For this review, take the finished solid that the model builds, in its own axes (mm). Face numbers are marked on the shaded views. A direction names the side the tool comes from. Give positions to 0.01 mm unless a question says otherwise; leave off trailing zeros. Order: outer loops, then holes, each group sorted by start corner. A loop starts at its lowest first (then second) coordinate and runs counter-clockwise, first axis right, second up.
Autodesk Inventor part; units mm, degrees
ref_plane "YZ Plane" through (0, 0, 0) normal (1, 0, 0) x (0, 1, 0)
ref_plane "XZ Plane" through (0, 0, 0) normal (0, 1, 0) x (-1, 0, 0)
ref_plane "XY Plane" through (0, 0, 0) normal (0, 0, 1) x (1, 0, 0)
sketch "Sketch1" plane through (0, 0, 0) normal (0, 0, 1) x (1, 0, 0)
  circle A0 centre (0, 0) radius 8.4
  circle A1 centre (0, 0) radius 11
  line L0 (9.5093, -0.878) -> (0, 0)
  line L1 (0, 0) -> (9.5093, 0.8821)
  line L2 (9.5093, 0.8821) -> (9.5093, -0.878)
  line L3 (0, 0) -> (-9.5093, 0.8821)
  line L4 (-9.5093, 0.8821) -> (-9.5093, -0.878)
  line L5 (-9.5093, -0.878) -> (0, 0)
  point P0 (8.3644, -0.7723)
  point P1 (-8.3644, -0.7723)
  point P2 (-8.3641, 0.7759)
  point P3 (8.3641, 0.7759)
  dimension "d0" = 16.8
  dimension "d1" = 22
extrude "Extrusion1" add sketch "Sketch1" along normal blind 15
sketch "Sketch2" plane through (0, 0, 15) normal (0, 0, 1) x (1, 0, 0)
  circle A0 centre (0, 0) radius 11
extrude "Extrusion2" add sketch "Sketch2" along normal blind 5
sketch "Sketch3" plane through (0, 0, 20) normal (0, 0, 1) x (1, 0, 0)
  line L0 (-5, 5) -> (5, 5)
  line L1 (5, 5) -> (5, -5)
  line L2 (5, -5) -> (-5, -5)
  line L3 (-5, -5) -> (-5, 5)
  line L4 (-5, 5) -> (5, -5) construction
  line L5 (5, 5) -> (-5, -5) construction
  point P0 (0, 0)
  dimension "d6" = 10
  dimension "d7" = 10
extrude "Extrusion3" add sketch "Sketch3" along normal blind 25
sketch "Sketch4" plane through (-5, 5, 20) normal (0, 1, 0) x (1, 0, 0)
  point P0 (5, 20)
sketch "Sketch5" plane through (-5, 5, 20) normal (0, 1, 0) x (1, 0, 0)
  line L0 (10, 0) -> (0, 0)
  line L1 (0, -25) -> (10, -25)
  line L2 (0, 0) -> (10, 0)
  line L3 (10, 0) -> (10, -25)
  line L4 (10, -25) -> (0, -25)
  line L5 (0, -25) -> (0, 0)
  point P0 (5, 20)
sketch "Sketch6" plane through (5, -5, 20) normal (1, 0, 0) x (0, 0, -1)
  line L0 (0, 10) -> (0, 0)
  line L1 (0, 0) -> (-25, 0)
  line L2 (0, 10) -> (-25, 10)
  line L3 (-25, 10) -> (-25, 0)
  line L4 (-25, 0) -> (0, 0)
  line L5 (0, 0) -> (0, 10)
  point P0 (20, 5)
extrude "Extrusion4" add sketch "Sketch6" along normal blind 20
extrude "Extrusion5" add sketch "Sketch5" along normal blind 20
mirror "Mirror1" about plane through (0, 0, 0) normal (0, 1, 0) of "Extrusion4", "Extrusion5"
mirror "Mirror2" about plane through (0, 0, 0) normal (1, 0, 0) of "Extrusion4"
sketch "Sketch7" plane through (25, 5, 20) normal (0, 0, -1) x (-1, 0, 0)
  line L0 (0, 0) -> (0, -10)
  arc A0 (20, 4.798) -> (15.202, 0) centre (25, -5) ccw
  line L1 (0, -10) -> (15.202, -10)
  line L2 (15.202, -10) -> (15.202, 0)
  line L3 (15.202, 0) -> (0, 0)
  line L4 (0, 0) -> (0, -10)
  arc A1 (15.202, 0) -> (15.202, -10) centre (25, -5) ccw
  circle A2 centre (25, -5) radius 11
  line L5 (20, -10) -> (20, -30)
  line L6 (30, -30) -> (30, -10)
  line L7 (20, -30) -> (30, -30)
  line L8 (30, -30) -> (30, -14.798)
  line L9 (30, -14.798) -> (20, -14.798)
  line L10 (20, -14.798) -> (20, -30)
  line L11 (30, 0) -> (30, 20)
  arc A3 (30, 4.798) -> (20, 4.798) centre (25, -5) ccw
  line L12 (30, 20) -> (20, 20)
  line L13 (20, 20) -> (20, 4.798)
  line L14 (20, 4.798) -> (30, 4.798)
  line L15 (30, 4.798) -> (30, 20)
  line L16 (30, 0) -> (50, 0)
  arc A4 (34.798, -10) -> (34.798, 0) centre (25, -5) ccw
  line L17 (50, 0) -> (34.798, 0)
  line L18 (34.798, 0) -> (34.798, -10)
  line L19 (34.798, -10) -> (50, -10)
  line L20 (50, -10) -> (50, 0)
  point P0 (30, 4.798)
extrude "Extrusion6" add sketch "Sketch7" along normal blind 20 contours L3 A1 L1 L0 | L13 L12 L11 A2 | A2 L6 L7 L5 | L16 L20 L19 A2
properties part number "2xxx_Rx_Coil_Winder_MPSv2_v1"
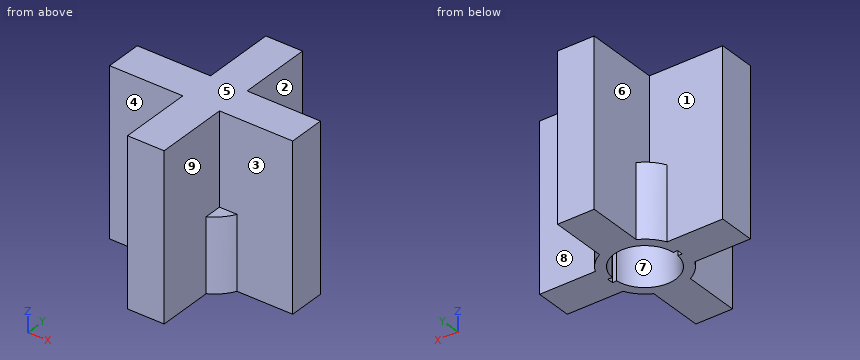
1) Clearance check with flat-ended pins moving along their axes: pin 1 (3 mm diameter, centred on y = -8.5, z = 17.5, fed in from +X); pin 2 (4 mm diameter, centred on y = -18.5, z = 37, fed in from +X); pin 3 (6 mm diameter, centred on x = -19, z = 17.5, fed in from +Y). State where each tip first meets the part, or that it passes through.
Answer sheet:
pin 1: stops at x = 8.49
pin 2: stops at x = 5
pin 3: stops at y = 5
2) We need section A-A on z = 24. Give the boundary of the cut face in (x, y), then the cut area to 3 significant figures.
Answer sheet:
outline: (-25, -5) - (-5, -5) - (-5, -25) - (5, -25) - (5, -5) - (25, -5) - (25, 5) - (5, 5) - (5, 25) - (-5, 25) - (-5, 5) - (-25, 5) - close
area: 900 mm2
3) We need section C-C on x = -7.5. Give the boundary of the cut face in (y, z).
Answer sheet:
outline: (-8.05, 0) - (-3.78, 0) - (-3.78, 15) - (3.78, 15) - (3.78, 0) - (8.05, 0) - (8.05, 20) - (5, 20) - (5, 45) - (-5, 45) - (-5, 20) - (-8.05, 20) - close
4) We need section D-D on z = 7. Give the boundary of the cut face in (x, y).
Answer sheet:
outline: (-25, -5) - (-9.8, -5) arc R11 ccw to (-5, -9.8) - (-5, -25) - (5, -25) - (5, -9.8) arc R11 ccw to (9.8, -5) - (25, -5) - (25, 5) - (9.8, 5) arc R11 ccw to (5, 9.8) - (5, 25) - (-5, 25) - (-5, 9.8) arc R11 ccw to (-9.8, 5) - (-25, 5) - close; hole (-9.51, -0.88) - (-8.36, -0.77) arc R8.4 ccw to (8.36, -0.77) - (9.51, -0.88) - (9.51, 0.88) - (8.36, 0.78) arc R8.4 ccw to (-8.36, 0.78) - (-9.51, 0.88) - close
5) To check wall thickness, follow line 1 (Y direction, x = 0.5, z = 10); line 2 (X direction, y = 0, z = 8); line 3 (X direction, y = 15.5, z = 11). State the ranges of each line that lie inside material, in increasing order.
Answer sheet:
line 1: y = -25 to -8.39, 8.39 to 25
line 2: x = -25 to -9.51, 9.51 to 25
line 3: x = -5 to 5
6) Tool access review of the marked faces 1, 2, 3, 4 and 5: name each direction out of +Z, -Z, +X, -X, +Y, -Y from which nothing blocks a thin tool from reaching the whole face with its end or side.
Answer sheet:
face 1: +Z, -X, +Y
face 2: +Z, +X, +Y
face 3: +Z, +X, -Y
face 4: +Z, -X, -Y
face 5: +Z, +X, -X, +Y, -Y
7) Draft analysis for pull direction X (two halves, no side actions). For the marked faces 6, 7, 8 and 9, state which applies: +X half, -X half, draft (parallel to the pull), parting line (faces both ways), or undercut.
Answer sheet:
face 6: -X half
face 7: undercut
face 8: draft
face 9: +X half
8) We need section B-B on y = 0. Give the boundary of the cut face in (x, z), then the cut area to 3 significant figures.
Answer sheet:
outline: (-25, 0) - (-9.51, 0) - (-9.51, 15) - (9.51, 15) - (9.51, 0) - (25, 0) - (25, 45) - (-25, 45) - close
area: 1,960 mm2
